from build123d import *

# Parameters (mm, degrees)
SKETCH2_R               = 20
SKETCH2_W               = 15
SKETCH2_H               = 30
BOSS_EXTRUDE1_DEPTH     = 30
FILLET1_R               = 17
CUT_EXTRUDE1_DEPTH      = 30
CUT_EXTRUDE1_DEPTH_BACK = 30
SKETCH3_W               = 15
SKETCH3_H               = 15
BOSS_EXTRUDE3_START     = 5
SKETCH4_R               = 20
BOSS_EXTRUDE3_DEPTH     = 5
SKETCH5_R               = 20
SKETCH5_R_2             = 18.5
CUT_EXTRUDE2_DEPTH      = 5
CUT_EXTRUDE3_DEPTH      = 20
CUT_EXTRUDE3_DEPTH_BACK = 40
SKETCH6_R               = 2.5


with BuildPart() as part:
    # Sketch2 → Boss-Extrude1 (new body)
    with BuildSketch(Plane(origin=(0, 0, 0), x_dir=(1, 0, 0), z_dir=(0, 1, 0))):
        with Locations(Location((0, 0, 0), (0, 0, 270))):
            Circle(SKETCH2_R)
        Rectangle(SKETCH2_W, SKETCH2_H, mode=Mode.SUBTRACT)
    extrude(amount=BOSS_EXTRUDE1_DEPTH)

    # Fillet1
    # the kernel refuses this fillet: 17 mm, written as the material it takes off along each edge
    with BuildSketch(Plane(origin=(0, 30, 0), x_dir=(0, 0, 1), z_dir=(-1, 0, 0))) as fillet1_piece_1:
        with BuildLine():
            CenterArc((20 - FILLET1_R, -FILLET1_R), FILLET1_R, 0, 90)
            Line((20 - FILLET1_R, 0), (20, 0))
            Line((20, 0), (20, -FILLET1_R))
        make_face()
    revolve(axis=Axis((0, 30, 0), (0, 1, 0)), mode=Mode.SUBTRACT)

    # Sketch3 → Cut-Extrude1 (cut, two sides: drawn at the far end of the back side and taken through both)
    with BuildSketch(Plane.XY.offset(-CUT_EXTRUDE1_DEPTH_BACK)):
        with Locations((0, 21.893596311)):
            Rectangle(SKETCH3_W, SKETCH3_H)
    extrude(amount=CUT_EXTRUDE1_DEPTH + CUT_EXTRUDE1_DEPTH_BACK, mode=Mode.SUBTRACT)

    # Sketch4 → Boss-Extrude3 (add)
    with BuildSketch(Plane.XZ.offset(BOSS_EXTRUDE3_START)):
        with Locations(Location((0, 0, 0), (0, 0, 270))):
            Circle(SKETCH4_R)
    extrude(amount=-BOSS_EXTRUDE3_DEPTH)

    # Sketch5 → Cut-Extrude2 (cut)
    with BuildSketch(Plane.XZ.offset(5)):
        with Locations(Location((0, 0, 0), (0, 0, 270))):
            Circle(SKETCH5_R)
        with Locations(Location((0, 0, 0), (0, 0, 270))):
            Circle(SKETCH5_R_2, mode=Mode.SUBTRACT)
    extrude(amount=-CUT_EXTRUDE2_DEPTH, mode=Mode.SUBTRACT)

    # Sketch6 → Cut-Extrude3 (cut, two sides: drawn at the far end of the back side and taken through both)
    with BuildSketch(Plane(origin=(0, 0, 0), x_dir=(0, 0, -1), z_dir=(1, 0, 0)).offset(-CUT_EXTRUDE3_DEPTH_BACK)):
        with Locations(Location((0, 22.393596311, 0), (0, 0, 310.060861392))):
            Circle(SKETCH6_R)
    extrude(amount=CUT_EXTRUDE3_DEPTH + CUT_EXTRUDE3_DEPTH_BACK, mode=Mode.SUBTRACT)


solid = part.part
Read the model definition and answer for the solid it produces. Units are mm, in the model's axes. A direction names the side the tool comes from. Coordinates: 2 decimals unless noted, no trailing zeros. One line per question, with ' | ' between items.
Q1. Find section A-A, the plane z = 0. State how many separate pieces and enclosed holes the cut face has, plus the area to 3 significant figures.
Result set:
separate pieces: 3 | enclosed holes: 0 | area: 717 mm^2
Q2. Consider L1, parallel to Z at x = 9, y = 21; L2, parallel to Y at x = 7, z = -7.5; L3, parallel to X at y = 0.5, z = -9. Determine where each line is inside the solid, lowest interval first. Write a range as [from, to].
Result set:
L1: [-15.59, -2.08], [2.08, 15.59] | L2: [-5, 0] | L3: [-17.86, -7.5], [7.5, 17.86]
Q3. Each of these flat-tipped pins is pushed along its axis until it touches: P1, Ø2, axis at x = -8.5, y = 20, coming from the -Z side; P2, Ø5, axis at x = -10.5, y = 12.5, coming from the +Z side; P3, Ø1.5, axis at x = 3.5, z = 11.5, coming from the +Y side; P4, Ø3, axis at y = 22.39, z = 0, coming from the +X side. Where does it stop, or does it pass through?
Result set:
P1: z = -17.1 | P2: z = 18.33 | P3: y = 0 | P4: through
Q4. For faces 1 (the flat face through (0, 14.394, 17)), 2 (the cylindrical face through (-7.086, -2.535, -17.089)), 3 (the flat face through (0, 0, 0)), determine the directions among +Z, -Z, +X, -X, +Y, -Y from which every point of the face is accessible in a straight line to the end or side of a thin tool.
Result set:
face 1: +Z, -Z, +Y | face 2: -Y | face 3: +Y
Q5. Determine the mould class of faces 4 (the flat face through (-7.5, 14, 0)), 5 (the flat face through (7.5, 14, 0)), 6 (the cylindrical face through (-19.524, 6.409, -4.336)), 7 (the flat face through (0, 14.394, -17)) for opening direction Z: +Z half, -Z half, draft (parallel to the pull), parting line (faces both ways), or undercut.
Result set:
face 4: undercut | face 5: undercut | face 6: parting line | face 7: draft
